Work out the finished part from the listing and answer in its coordinate system (mm). A direction names the side the tool comes from. Coordinates: 2 decimals unless noted, no trailing zeros. Write each loop counter-clockwise with the first axis right and the second up, starting at its lowest first coordinate (ties: lowest second). Pieces come first, ordered by that corner, then holes. Notation, with made-up numbers: (77, 1.5) - (102, 1.5) arc R13 cw to (102, 21.5) - close; hole circle Ø8 at (67, -17.5). An arc over 180 degrees is marked (long way). Use a Markdown table: item, result. Add a question column.
(1) A tool of negligible diameter and unlimited length cuts with its end or side. For faces 4 (the face through (0, 2, -13.5)), 5 (the face through (19.989, 1, 0)), 6 (the face through (-34, 2, 13.5)), 7 (the face through (-34, 2, -13.5)), 8 (the face through (34, 2, 13.5)), from which of +Z, -Z, +X, -X, +Y, -Y can it reach the whole face along a straight path? Write none if from no direction.
(2) Given pin 1 Ø1.2 at (x, z) = (-19.76, 18.26) entering from +Y; pin 2 Ø1.8 at (x, y) = (7, 1) entering from +Z; pin 3 Ø12 at (x, z) = (25.5, -6) entering from +Y, each flat-ended and moving along its own axis, determine where each tip first touches the part or whether it passes through.
(3) The part is cut by section B-B, the plane y = 0.65. Give the vertices of the cut face in (x, z), then the cut area to 3 significant figures.
(4) For a pull along X with two mould halves and no side action, classify faces 1 (the face through (-28, 2.5, 0)), 2 (the face through (0.535, 2.993, -33.167)), 3 (the face through (0, 2, 13.5)) as released by +X, released by -X, zero draft, split by the parting line, or undercut.
(5) Find the intervals of material crossed by line 1 (X direction, y = 0.5, z = 13); line 2 (Z direction, x = -19, y = 2.3); line 3 (Y direction, x = 22.5, z = 9), in increasing order. Write a range as from..to.
(6) The part is cut by section A-A, the plane z = -4.5. Give the vertices of the cut face in (x, y), then the cut area to 3 significant figures.
from build123d import *

# Parameters (mm, degrees)
SKETCH7_R           = 33.17091481
BOSS_EXTRUDE2_DEPTH = 1
SKETCH13_W          = 75
SKETCH13_H          = 27
CUT_EXTRUDE2_DEPTH  = 54.148377209
SKETCH18_W          = 14.996875164
SKETCH18_H          = 27
BOSS_EXTRUDE4_DEPTH = 2.5
SKETCH18_3_W        = 14.996875164
SKETCH18_3_H        = 27
SKETCH18_3_W_2      = 14.998441489
BOSS_EXTRUDE5_DEPTH = 2.5
SKETCH20_R          = 0.999251596
SKETCH20_R_2        = 1.000371823
CUT_EXTRUDE3_DEPTH  = 52.40525265


with BuildPart() as part:
    # Sketch3 → Revolve1 (revolve)
    with BuildSketch(Plane.XY, mode=Mode.PRIVATE) as revolve1_sk:
        Polygon((0, 0), (37.5, 0), (33.17091481, 2.5), (0, 2.5), align=None)
    revolve(revolve1_sk.sketch.rotate(Axis((0, 0, 0), (0, 1, 0)), 90), axis=Axis((0, 0, 0), (0, 1, 0)))

    # Sketch7 → Boss-Extrude2 (add)
    with BuildSketch(Plane(origin=(0, 2.5, 0), x_dir=(1, 0, 0), z_dir=(0, 1, 0))):
        with Locations(Location((0, 0, 0), (0, 0, 270))):
            Circle(SKETCH7_R)
    extrude(amount=BOSS_EXTRUDE2_DEPTH)

    # Sketch13 → Cut-Extrude2 (cut, through all)
    with BuildSketch(Plane.XZ):
        Rectangle(SKETCH13_W, SKETCH13_H)
    extrude(amount=-CUT_EXTRUDE2_DEPTH, mode=Mode.SUBTRACT)


with BuildPart() as cut_extrude2_piece_1:
    # of the separate pieces the step leaves, piece 1, a body of its own (cut_extrude2_pieces)
    add(part.part.solids().sort_by_distance((-34.985711369, 0, -13.5))[0])



with BuildPart() as cut_extrude2_piece_2:
    # of the separate pieces the step leaves, piece 2, a body of its own (cut_extrude2_pieces)
    add(part.part.solids().sort_by_distance((-34.985711369, 0, 13.5))[0])


with BuildPart() as cut_extrude2_piece_1_1:
    add(cut_extrude2_piece_1.part)

    add(cut_extrude2_piece_2.part)  # Boss-Extrude4 merges Cut-Extrude2 piece 2
    # Sketch18 → Boss-Extrude4 (add)
    with BuildSketch(Plane(origin=(0, 0, 0), x_dir=(1, 0, 0), z_dir=(0, 1, 0))):
        with Locations((27.487273787, 0)):
            Rectangle(SKETCH18_W, SKETCH18_H)
    extrude(amount=BOSS_EXTRUDE4_DEPTH)

    # Sketch18_3 → Boss-Extrude5 (add)
    with BuildSketch(Plane(origin=(0, 0, 0), x_dir=(1, 0, 0), z_dir=(0, 1, 0))):
        with Locations((27.487273787, 0)):
            Rectangle(SKETCH18_3_W, SKETCH18_3_H)
        with Locations((-27.486490625, 0)):
            Rectangle(SKETCH18_3_W_2, SKETCH18_3_H)
    extrude(amount=BOSS_EXTRUDE5_DEPTH)

    # Sketch20 → Cut-Extrude3 (cut, through all)
    with BuildSketch(Plane(origin=(0, 3.5, 0), x_dir=(1, 0, 0), z_dir=(0, 1, 0))):
        with Locations(Location((-19.757076847, -18.256562674, 0), (0, 0, 270))):
            Circle(SKETCH20_R)
        with Locations(Location((20.497529554, 18.200406752, 0), (0, 0, 270))):
            Circle(SKETCH20_R_2)
    extrude(amount=-CUT_EXTRUDE3_DEPTH, mode=Mode.SUBTRACT)


solid = cut_extrude2_piece_1_1.part
Model answer:
| question | item | result |
|---|---|---|
| 1 | face 4 | +Y |
| 1 | face 5 | +Y, -Y |
| 1 | face 6 | +Z, -X, +Y |
| 1 | face 7 | -Z, -X, +Y |
| 1 | face 8 | +Z, +X, +Y |
| 2 | pin 1 | through |
| 2 | pin 2 | z = 36.67 |
| 2 | pin 3 | y = 2.5 |
| 3 | outline | (-34.99, -13.5) - (-33.78, -13.5) arc R36.37 ccw to (33.78, -13.5) - (34.99, -13.5) - (34.99, 13.5) - (33.78, 13.5) arc R36.37 ccw to (-33.78, 13.5) - (-34.99, 13.5) - close; hole circle Ø2 at (-19.76, 18.26); hole (-19.99, -13.5) - (19.99, -13.5) - (19.99, 13.5) - (-19.99, 13.5) - close; hole circle Ø2 at (20.5, -18.2) |
| 3 | area | 3,040 mm^2 |
| 4 | face 1 | zero draft |
| 4 | face 2 | split by the parting line |
| 4 | face 3 | undercut |
| 5 | line 1 | -34.99..-19.99, 19.99..34.99 |
| 5 | line 2 | -27.61..-13.5, 13.5..17.6, 18.91..27.61 |
| 5 | line 3 | 0..2.5 |
| 6 | outline | (-34.99, 0) - (-19.99, 0) - (-19.99, 2.5) - (-34.99, 2.5) - close; (19.99, 0) - (34.99, 0) - (34.99, 2.5) - (19.99, 2.5) - close |
| 6 | area | 75.0 mm^2 |
